Check sheet for the drawn part. Datum: minimum x, y, z corner. Units: mm. A direction names the side the tool comes from. Coordinates: 2 decimals unless noted, no trailing zeros. Write each loop counter-clockwise with the first axis right and the second up, starting at its lowest first coordinate (ties: lowest second). Pieces come first, ordered by that corner, then holes. Notation, with made-up numbers: (-7, 72) - (47, 72) arc R20 cw to (47, 102) - close; hole circle Ø8 at (-8.75, -31). An arc over 180 degrees is marked (long way). Write each question's results on one line, items separated by ' | '.
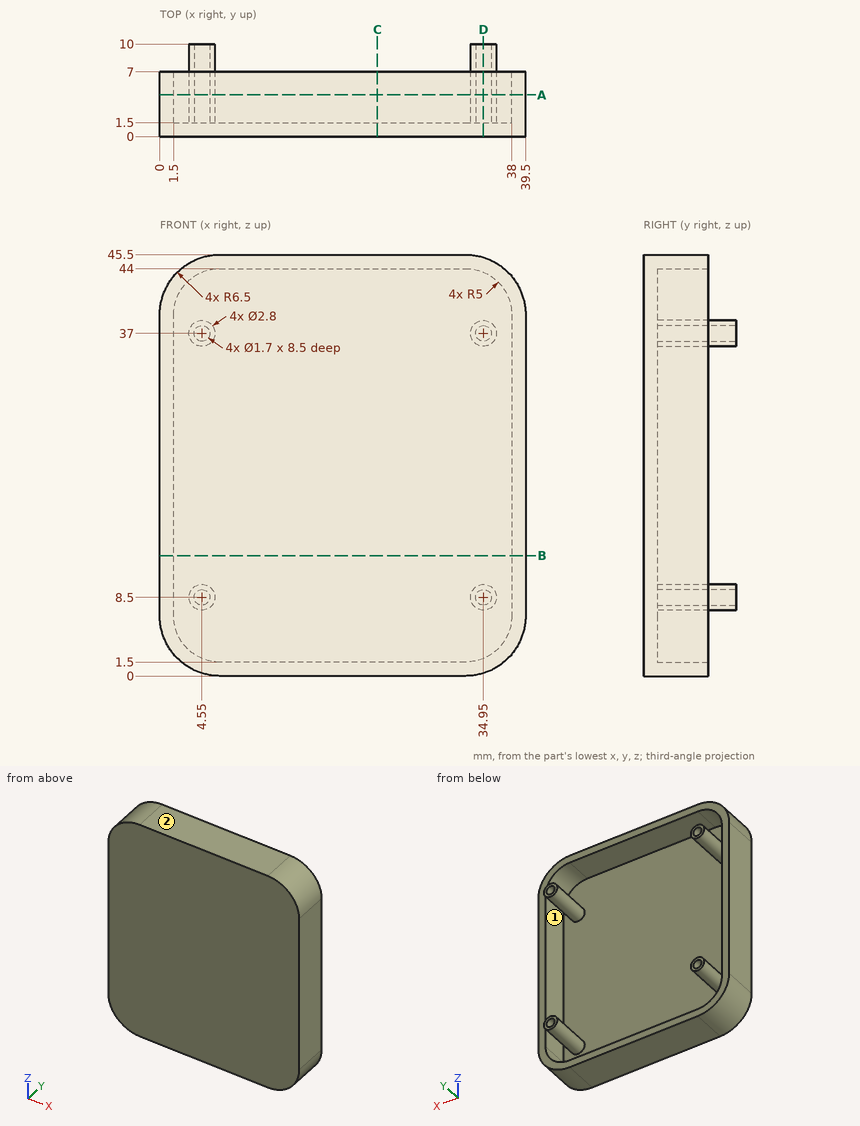
1. Sectioned sample at D-D (x = 34.95). Record the cut outline in (y, z).
Values follow:
outline: (0, 0.3) - (7, 0.3) - (7, 1.9) - (1.5, 1.9) - (1.5, 7.1) - (10, 7.1) - (10, 7.65) - (1.5, 7.65) - (1.5, 9.35) - (10, 9.35) - (10, 9.9) - (1.5, 9.9) - (1.5, 35.6) - (10, 35.6) - (10, 36.15) - (1.5, 36.15) - (1.5, 37.85) - (10, 37.85) - (10, 38.4) - (1.5, 38.4) - (1.5, 43.6) - (7, 43.6) - (7, 45.2) - (0, 45.2) - close
2. Sectioned sample at C-C (x = 23.5). Record the cut outline in (y, z).
Values follow:
outline: (0, 0) - (7, 0) - (7, 1.5) - (1.5, 1.5) - (1.5, 44) - (7, 44) - (7, 45.5) - (0, 45.5) - close
3. Material ranges on L1, parallel to X at y = 6, z = 37; L2, parallel to X at y = 8.5, z = 37; L3, parallel to Z at x = 28, y = 6, recorded low to high. Write a range as [from, to].
Values follow:
L1: x = [0, 1.5], [3.15, 3.7], [5.4, 5.95], [33.55, 34.1], [35.8, 36.35], [38, 39.5] | L2: x = [3.15, 3.7], [5.4, 5.95], [33.55, 34.1], [35.8, 36.35] | L3: z = [0, 1.5], [44, 45.5]
4. Access from +Z, -Z, +X, -X, +Y, -Y to the whole of each face (thin tool, end or side, straight path). Record for the marked faces 1 and 2.
Values follow:
face 1: +Y | face 2: +Z, +X, -X, +Y, -Y
5. Sectioned sample at B-B (z = 13). Record the cut outline in (x, y).
Values follow:
outline: (0, 0) - (39.5, 0) - (39.5, 7) - (38, 7) - (38, 1.5) - (1.5, 1.5) - (1.5, 7) - (0, 7) - close
6. Sectioned sample at A-A (y = 4.5). Give the number of separate pieces and of enclosed holes in the cut face, then the cut area to 3 significant figures.
Values follow:
separate pieces: 5 | enclosed holes: 5 | area: 247 mm^2
7. Go/stop test with a flat-tipped pin: pin 1 (0.5 mm diameter, centred on x = 35, z = 8.5, fed in from +Y). Record where the tip stops, or that it passes through.
Values follow:
pin 1: stops at y = 1.5
